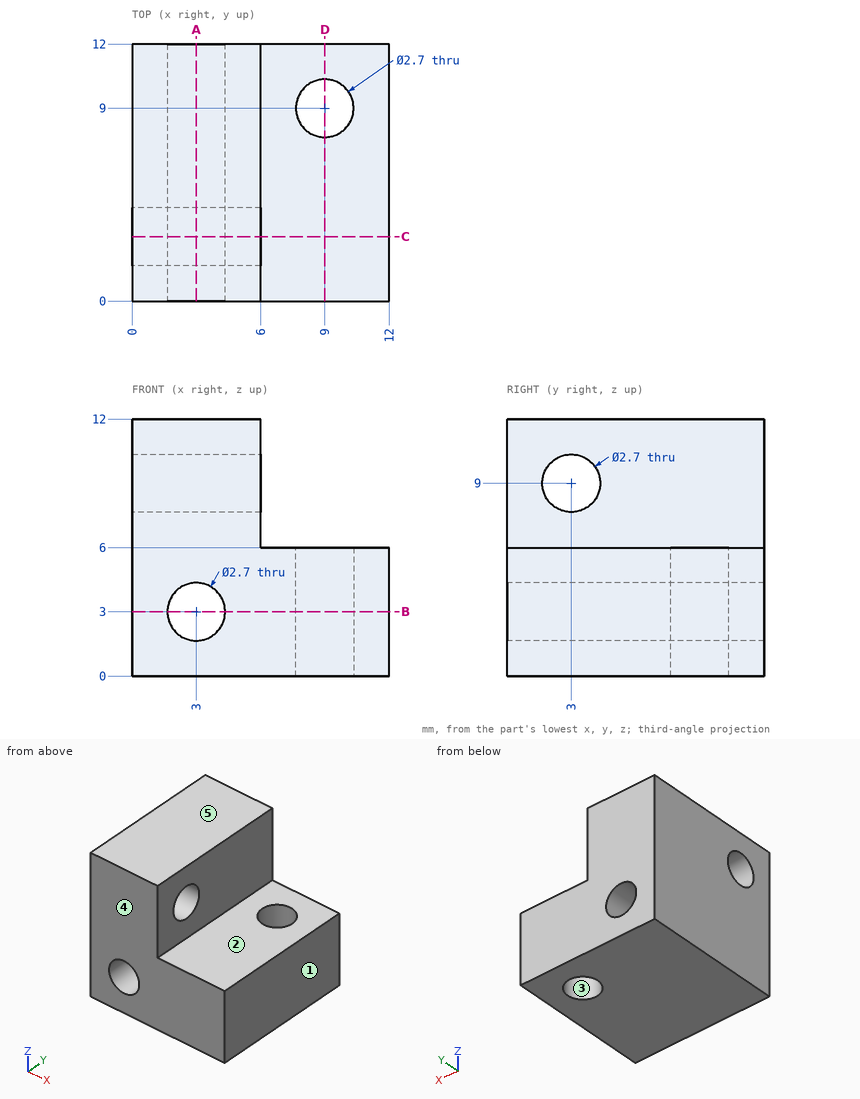
Here's the drawing with two shaded views (mm, measured from the low corner). I have some questions. A direction names the side the tool comes from. Coordinates: 2 decimals unless noted, no trailing zeros. Loops run counter-clockwise (first coordinate to the right, second up) from the corner with the lowest first, then second, coordinate; pieces in that order, holes last. Notation, with made-up numbers: M 41.5,60 L 88.5,60 A4 cw 88.5,64 Z; hole C 40.25,70 d8. An arc over 180 degrees is marked long. Return JSON: item names as keys, results as strings. Group by question number.
Item 1: I'm going to push flat-ended pins straight in: pin 1 Ø5 at (y, z) = (7.5, 10) entering from +X; pin 2 Ø1 at (x, z) = (9.5, 7.5) entering from +Y; pin 3 Ø1.8 at (x, y) = (9, 3.5) entering from +Z. Where does each tip first touch, or does it pass through?
Item 2: On a 3-axis mill with a long thin cutter (end or side, diameter ignored), from which of +Z, -Z, +X, -X, +Y, -Y can I reach the whole of each face in a straight line? I mean the marked faces 1 and 2. Say none if no direction works.
Item 3: Thinking about a two-plate mould opening in Y: for the marked faces 3, 4 and 5, which applies, released by +Y, released by -Y, zero draft, split by the parting line, or undercut?
Item 4: If I drill on L1, parallel to Z at x = 3, y = 6; L2, parallel to Y at x = 9, z = 3.75; L3, parallel to X at y = 2.75, z = 7.5, over which ranges is the centre line in solid material (lowest first)? Write a range as from..to.
Item 5: Imagine slicing it at B-B (z = 3). Please give me the cut outline in (x, y), and give its area (3 significant figures).
Item 6: Imagine slicing it at C-C (y = 3). Please give me the cut outline in (x, z).
Item 7: Imagine slicing it at D-D (x = 9). Please give me the cut outline in (y, z), and give its area (3 significant figures).
Item 8: Imagine slicing it at A-A (x = 3). Please give me the cut outline in (y, z).
Verdict:
{
 "1": {"pin 1": "stops at x = 6", "pin 2": "passes through", "pin 3": "stops at z = 6"},
 "2": {"face 1": "+Z, -Z, +X, +Y, -Y", "face 2": "+Z, +X, +Y, -Y"},
 "3": {"face 3": "undercut", "face 4": "released by -Y", "face 5": "zero draft"},
 "4": {"L1": "z = 0..1.65, 4.35..12", "L2": "y = 0..7.65, 10.35..12", "L3": "x = 0..6"},
 "5": {"outline": "M 0,0 L 1.65,0 L 1.65,12 L 0,12 Z; M 4.35,0 L 12,0 L 12,12 L 4.35,12 Z; hole C 9,9 d2.7", "area": "106 mm^2"},
 "6": {"outline": "M 0,0 L 12,0 L 12,6 L 6,6 L 6,7.65 L 0,7.65 Z; M 0,10.35 L 6,10.35 L 6,12 L 0,12 Z; hole C 3,3 d2.7"},
 "7": {"outline": "M 0,0 L 7.65,0 L 7.65,6 L 0,6 Z; M 10.35,0 L 12,0 L 12,6 L 10.35,6 Z", "area": "55.8 mm^2"},
 "8": {"outline": "M 0,0 L 12,0 L 12,1.65 L 0,1.65 Z; M 0,4.35 L 12,4.35 L 12,12 L 0,12 Z; hole C 3,9 d2.7"}
}
